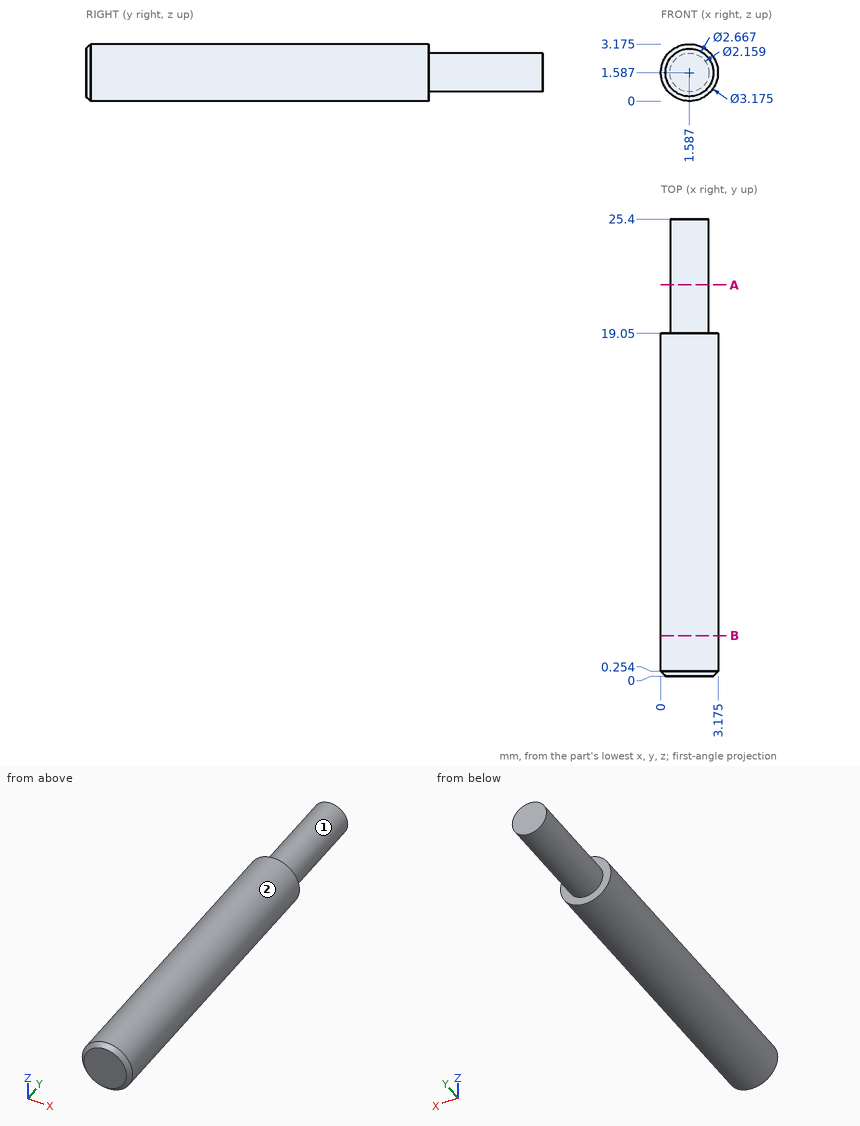
Geometry check sheet. Reference: drawing and pictorial views, mm from the part's lowest x, y, z. A direction names the side the tool comes from. Give positions to 0.01 mm unless a question says otherwise; leave off trailing zeros. Order: outer loops, then holes, each group sorted by start corner. A loop starts at its lowest first (then second) coordinate and runs counter-clockwise, first axis right, second up. Notation, with made-up numbers: (34.5, 15) -> (84.5, 15) arc R29 cw to (84.5, 35) -> close; hole circle Ø11 at (89.25, 8.25). An arc over 180 degrees is marked (long way). Write each question's results on one line, items separated by ' | '. Start each with the question number.
(1) Gauge pin test, flat end, axial feed: P1, Ø1, axis at y = 5, z = 2.5, coming from the -X side (1 decimal). Record the tip position at first contact, or that the pin passes through.
(2) Sectioned sample at A-A (y = 21.75). Enter the section's corners in (x, z).
(3) Scan lines: line 1 (X direction, y = 11, z = 2.45) (1 decimal); line 2 (X direction, y = 22.25, z = 1.55); line 3 (Z direction, x = 0.5, y = 15.5) (1 decimal). Record each from-to range of solid material in increasing order.
(4) Access from +Z, -Z, +X, -X, +Y, -Y to the whole of each face (thin tool, end or side, straight path). Record for the marked faces 1 and 2.
(5) Sectioned sample at B-B (y = 2.25). Enter the section's corners in (x, z) (1 decimal).
Answer below:
1) P1: x = 0.1
2) outline: circle Ø2.16 at (1.59, 1.59)
3) line 1: 0.3 to 2.9 | line 2: 0.51 to 2.67 | line 3: 0.4 to 2.7
4) face 1: +Y | face 2: +Y, -Y
5) outline: circle Ø3.2 at (1.6, 1.6)
